from build123d import *

# Parameters (mm, degrees)
EXTRUDE_1_DEPTH          = 33
CUT_EXTRUDE_1_DEPTH      = 186.485848517
CUT_EXTRUDE_1_DEPTH_BACK = 186.485848517
SKETCH_2_R               = 6


with BuildPart() as part:
    # Эскиз1 → Бобышка-Вытянуть1 (new body)
    with BuildSketch(Plane.XY):
        with BuildLine():
            Line((0, 0), (38, 0))
            ThreePointArc((38, 0), (47.899494937, 4.100505063), (52, 14))
            Line((52, 14), (52, 150))
            Line((52, 150), (48, 150))
            Line((48, 150), (48, 14))
            ThreePointArc((48, 14), (45.071067812, 6.928932188), (38, 4))
            Line((38, 4), (0, 4))
            Line((0, 4), (-38, 4))
            ThreePointArc((-38, 4), (-45.071067812, 6.928932188), (-48, 14))
            Line((-48, 14), (-48, 150))
            Line((-48, 150), (-52, 150))
            Line((-52, 150), (-52, 14))
            ThreePointArc((-52, 14), (-47.899494937, 4.100505063), (-38, 0))
            Line((-38, 0), (0, 0))
        make_face()
    extrude(amount=EXTRUDE_1_DEPTH)

    # Эскиз2 → Вырез-Вытянуть1 (cut, two sides: drawn at the far end of the back side and taken through both)
    with BuildSketch(Plane(origin=(52, 0, 0), x_dir=(0, 0, -1), z_dir=(1, 0, 0)).offset(-CUT_EXTRUDE_1_DEPTH_BACK)):
        with Locations((-16.5, 124)):
            Circle(SKETCH_2_R)
    extrude(amount=CUT_EXTRUDE_1_DEPTH + CUT_EXTRUDE_1_DEPTH_BACK, mode=Mode.SUBTRACT)


solid = part.part
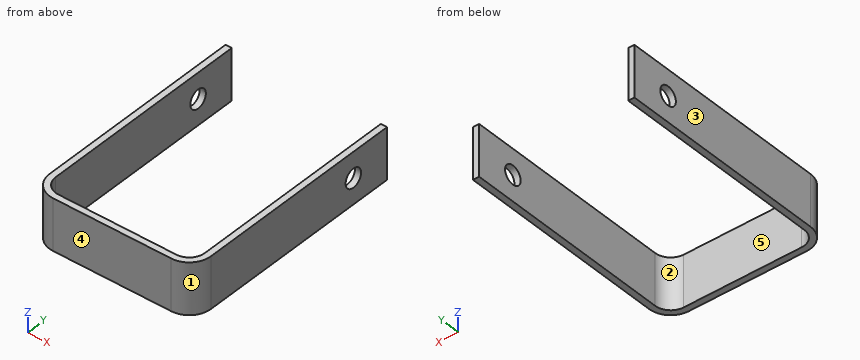
Could you check a few things on this model? Use its own coordinates, in mm. Face numbers are marked on the shaded views. A direction names the side the tool comes from. Give positions to 0.01 mm unless a question says otherwise; leave off trailing zeros. Loops run counter-clockwise (first coordinate to the right, second up) from the corner with the lowest first, then second, coordinate; pieces in that order, holes last. Notation, with made-up numbers: (10, 72) -> (62, 72) arc R35 cw to (62, 111) -> close; hole circle Ø4 at (30, 16.5). An arc over 180 degrees is marked (long way). Return JSON: item names as keys, results as strings.
Item 1: Which directions (+Z, -Z, +X, -X, +Y, -Y) give clear straight access to the entire face, cutting with the end or side of a thin tool? Please do the marked faces 4 and 5.
Geometry results:
{"face 4": "+Z, -Z, +X, -X, -Y", "face 5": "+Z, -Z, +Y"}
Item 2: We'd pull the mould along X, two halves only. Please class the marked faces 1, 2 and 3: +X half, -X half, draft (parallel to the pull), parting line (faces both ways), or undercut.
Geometry results:
{"face 1": "+X half", "face 2": "undercut", "face 3": "-X half"}
Item 3: If we section it at C-C on y = 124: List the corners of the cut face in (x, z) for me, plus the area to 3 significant figures.
Geometry results:
{"outline": "(-52, 0) -> (-48, 0) -> (-48, 10.5) -> (-52, 10.5) -> close; (-52, 22.5) -> (-48, 22.5) -> (-48, 33) -> (-52, 33) -> close; (48, 0) -> (52, 0) -> (52, 10.5) -> (48, 10.5) -> close; (48, 22.5) -> (52, 22.5) -> (52, 33) -> (48, 33) -> close", "area": "168 mm²"}
Item 4: I'm going to push flat-ended pins straight in: pin 1 (1 mm diameter, centred on x = 29.5, z = 11.5, fed in from +Y); pin 2 (9.5 mm diameter, centred on y = 124, z = 16.5, fed in from +X) (1 decimal). Where does each tip first touch, or does it pass through?
Geometry results:
{"pin 1": "stops at y = 4", "pin 2": "passes through"}
Item 5: If we section it at D-D on x = -18.5: List the corners of the cut face in (y, z) for me.
Geometry results:
{"outline": "(0, 0) -> (4, 0) -> (4, 33) -> (0, 33) -> close"}
Item 6: I need wall thicknesses on L1, parallel to X at y = 38.5, z = 7.5; L2, parallel to Z at x = -50.3, y = 124; L3, parallel to Y at x = 2, z = 1.5. Which ranges of each line are inside material? Lowest first, please. Write a range as from..to.
Geometry results:
{"L1": "x = -52..-48, 48..52", "L2": "z = 0..10.5, 22.5..33", "L3": "y = 0..4"}
Item 7: If we section it at A-A on y = 93: List the corners of the cut face in (x, z) for me.
Geometry results:
{"outline": "(-52, 0) -> (-48, 0) -> (-48, 33) -> (-52, 33) -> close; (48, 0) -> (52, 0) -> (52, 33) -> (48, 33) -> close"}
Item 8: If we section it at B-B on z = 16.5: List the corners of the cut face in (x, y) for me.
Geometry results:
{"outline": "(-52, 14) arc R14 ccw to (-38, 0) -> (38, 0) arc R14 ccw to (52, 14) -> (52, 118) -> (48, 118) -> (48, 14) arc R10 cw to (38, 4) -> (-38, 4) arc R10 cw to (-48, 14) -> (-48, 118) -> (-52, 118) -> close; (-52, 130) -> (-48, 130) -> (-48, 150) -> (-52, 150) -> close; (48, 130) -> (52, 130) -> (52, 150) -> (48, 150) -> close"}
